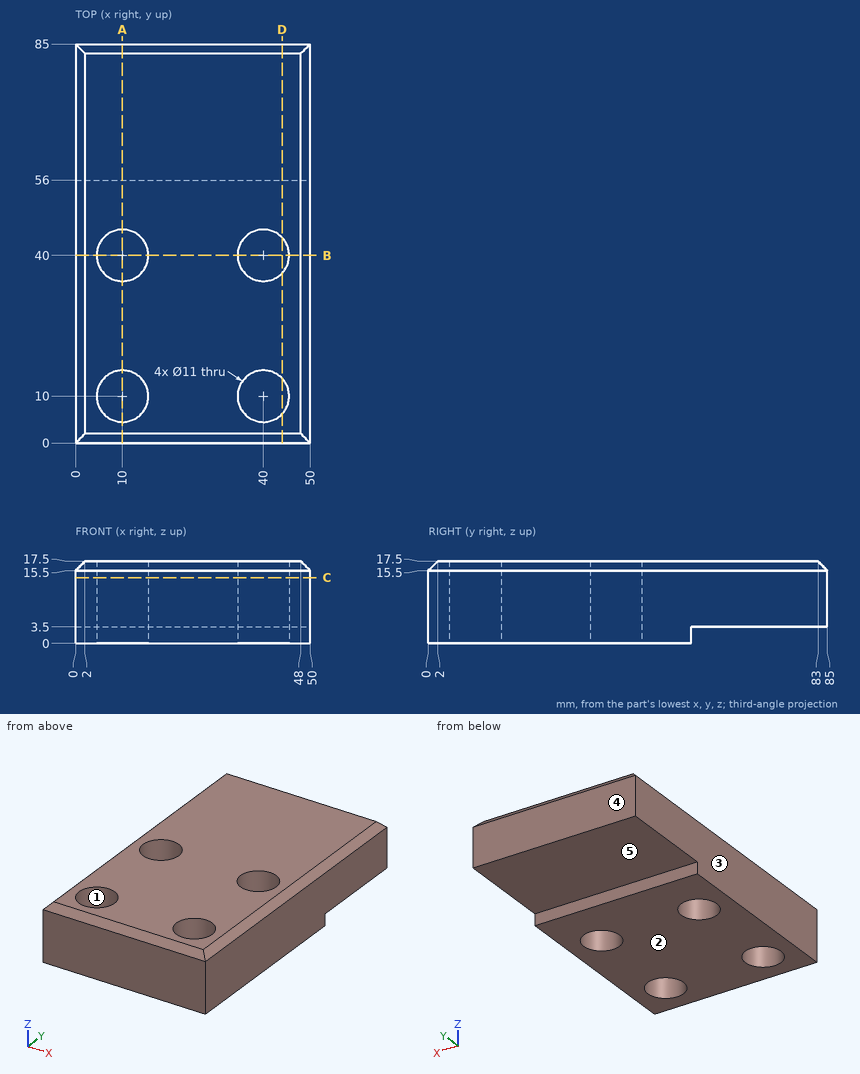
Design review of the part shown in the three views and the two pictorial views. Dimensions are in mm from the part's minimum x, y and z. A direction names the side the tool comes from. Give positions to 0.01 mm unless a question says otherwise; leave off trailing zeros. Write each loop counter-clockwise with the first axis right and the second up, starting at its lowest first coordinate (ties: lowest second). Pieces come first, ordered by that corner, then holes.
Item 1: The part is to be moulded in two halves that separate along X. For the marked faces 1, 2 and 3, say which applies: +X half, -X half, draft (parallel to the pull), parting line (faces both ways), or undercut.
Item 2: Take a section at A-A (x = 10). Give the boundary of the cut face in (y, z).
Item 3: Take a section at D-D (x = 44). Give the boundary of the cut face in (y, z).
Item 4: Machinability: for the marked faces 4 and 5, which of the approach directions +Z, -Z, +X, -X, +Y, -Y give a long, thin tool a straight path to every point of the face, cutting with its end or side? Answer none if there is none.
Item 5: Take a section at C-C (z = 14). Give the boundary of the cut face in (x, y).
Item 6: Insertion check: P1, Ø5, axis at y = 70, z = 2.5, coming from the -X side; P2, Ø1.8, axis at x = 20, z = 2, coming from the +Y side; P3, Ø10, axis at x = 10, y = 10, coming from the +Z side. Each pin has a flat end and moves straight along its axis. Give the tip position at first contact, or say it passes through.
Item 7: Take a section at B-B (y = 40). Give the boundary of the cut face in (x, z).
Item 8: Wall thickness on probe 1 along Y at (x, z) = (40, 6.5); probe 2 along X at (y, z) = (11.5, 14); probe 3 along X at (y, z) = (15, 16.25): over which ranges is each line inside the solid? List them lowest first.
Established:
1. face 1: undercut
1. face 2: draft
1. face 3: -X half
2. outline: (0, 0) - (4.5, 0) - (4.5, 17.5) - (2, 17.5) - (0, 15.5) - close; (15.5, 0) - (34.5, 0) - (34.5, 17.5) - (15.5, 17.5) - close; (45.5, 0) - (56, 0) - (56, 3.5) - (85, 3.5) - (85, 15.5) - (83, 17.5) - (45.5, 17.5) - close
3. outline: (0, 0) - (6.23, 0) - (6.23, 17.5) - (2, 17.5) - (0, 15.5) - close; (13.77, 0) - (36.23, 0) - (36.23, 17.5) - (13.77, 17.5) - close; (43.77, 0) - (56, 0) - (56, 3.5) - (85, 3.5) - (85, 15.5) - (83, 17.5) - (43.77, 17.5) - close
4. face 4: +Z, -Z, +X, -X, +Y
4. face 5: -Z, +X, -X, +Y
5. outline: (0, 0) - (50, 0) - (50, 85) - (0, 85) - close; hole circle Ø11 at (10, 10); hole circle Ø11 at (10, 40); hole circle Ø11 at (40, 10); hole circle Ø11 at (40, 40)
6. P1: stops at x = 0
6. P2: stops at y = 56
6. P3: passes through
7. outline: (0, 0) - (4.5, 0) - (4.5, 17.5) - (2, 17.5) - (0, 15.5) - close; (15.5, 0) - (34.5, 0) - (34.5, 17.5) - (15.5, 17.5) - close; (45.5, 0) - (50, 0) - (50, 15.5) - (48, 17.5) - (45.5, 17.5) - close
8. probe 1: y = 0 to 4.5, 15.5 to 34.5, 45.5 to 85
8. probe 2: x = 0 to 4.71, 15.29 to 34.71, 45.29 to 50
8. probe 3: x = 0.75 to 7.71, 12.29 to 37.71, 42.29 to 49.25
